Could you check a few things on this model? Use its own coordinates, in mm. Face numbers are marked on the shaded views. A direction names the side the tool comes from. Round coordinates to 2 decimals unless told otherwise and drop trailing zeros. Order: outer loops, then holes, each group sorted by start corner. A loop starts at its lowest first (then second) coordinate and runs counter-clockwise, first axis right, second up. Notation, with made-up numbers: (-3, 74) - (11, 74) arc R18 ccw to (11, 100) - close; hole circle Ø3 at (64, -7.5). An arc over 180 degrees is marked (long way). Use one line per item in the form item = value.
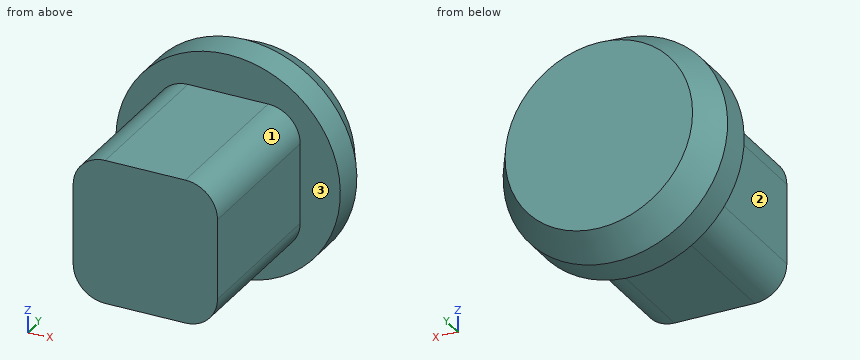
from build123d import *

# Parameters (mm, degrees)
SKETCH_2_W      = 4.5
SKETCH_2_H      = 4.5
EXTRUDE_1_DEPTH = 5
SKETCH_3_R      = 3.5
EXTRUDE_2_DEPTH = 2
CHAMFER_1_SIZE  = 1
CHAMFER_1_SIZE2 = 0.577350269
FILLET_1_R      = 1


with BuildPart() as part:
    # Эскиз2 → Бобышка-Вытянуть1 (new body)
    with BuildSketch(Plane(origin=(0, 0, 0), x_dir=(1, 0, 0), z_dir=(0, 1, 0))):
        Rectangle(SKETCH_2_W, SKETCH_2_H)
    extrude(amount=EXTRUDE_1_DEPTH)

    # Эскиз3 → Бобышка-Вытянуть2 (add)
    with BuildSketch(Plane(origin=(0, 5, 0), x_dir=(1, 0, 0), z_dir=(0, 1, 0))):
        with Locations(Location((0, 0, 0), (0, 0, 270))):
            Circle(SKETCH_3_R)
    extrude(amount=EXTRUDE_2_DEPTH)

    # Фаска1
    chamfer_1_edges = [part.edges().sort_by_distance(p)[0] for p in [
        (0, 7, -3.5),
    ]]
    chamfer_1_side = [part.faces().sort_by_distance(p)[0] for p in [
        (0, 6, -3.5),
    ]]
    chamfer(chamfer_1_edges, length=CHAMFER_1_SIZE, length2=CHAMFER_1_SIZE2, reference=chamfer_1_side[0])

    # Скругление1
    fillet_1_edges = [part.edges().sort_by_distance(p)[0] for p in [
        (2.25, 2.5, 2.25),
        (-2.25, 2.5, 2.25),
        (-2.25, 2.5, -2.25),
        (2.25, 2.5, -2.25),
    ]]
    fillet(fillet_1_edges, radius=FILLET_1_R)


solid = part.part
Item 1: I need wall thicknesses on L1, parallel to Y at x = 2.5, z = -0.25; L2, parallel to X at y = 1.25, z = 0. Which ranges of each line are inside material? Lowest first, please.
Found:
L1 = 5 to 7
L2 = -2.25 to 2.25
Item 2: Imagine slicing it at D-D on y = 5.5. Please give me the cut outline in (x, z).
Found:
outline = circle Ø7 at (0, 0)
Item 3: For the marked faces 1, 2 and 3, which set-ups out of +Z, -Z, +X, -X, +Y, -Y let a thin tool reach every point of the face, with its end or its side?
Found:
face_1 = +Z, +X, -Y
face_2 = +Z, -Z, -X, -Y
face_3 = -Y
Item 4: Imagine slicing it at B-B on z = 0. Please give me the cut outline in (x, y), plus the area to 3 significant figures.
Found:
outline = (-3.5, 5) - (-2.25, 5) - (-2.25, 0) - (2.25, 0) - (2.25, 5) - (3.5, 5) - (3.5, 6) - (2.92, 7) - (-2.92, 7) - (-3.5, 6) - close
area = 35.9 mm2
Item 5: Imagine slicing it at A-A on y = 4.75. Please give me the cut outline in (x, z), plus the area to 3 significant figures.
Found:
outline = (-2.25, -1.25) arc R1 ccw to (-1.25, -2.25) - (1.25, -2.25) arc R1 ccw to (2.25, -1.25) - (2.25, 1.25) arc R1 ccw to (1.25, 2.25) - (-1.25, 2.25) arc R1 ccw to (-2.25, 1.25) - close
area = 19.4 mm2
Item 6: Will these pins go through, and if not, where does the flat tip stop? P1, Ø1.3, axis at x = 0.5, y = 2, coming from the -Z side; P2, Ø0.8, axis at y = 3, z = -0.5, coming from the +X side; P3, Ø2, axis at x = 0.5, y = 1.5, coming from the +Z side; P4, Ø1.5, axis at x = -0.5, z = -1, coming from the -Y side.
Found:
P1 = -2.25
P2 = 2.25
P3 = 2.25
P4 = 0
Item 7: Imagine slicing it at C-C on x = 0. Please give me the cut outline in (y, z).
Found:
outline = (0, -2.25) - (5, -2.25) - (5, -3.5) - (6, -3.5) - (7, -2.92) - (7, 2.92) - (6, 3.5) - (5, 3.5) - (5, 2.25) - (0, 2.25) - close
